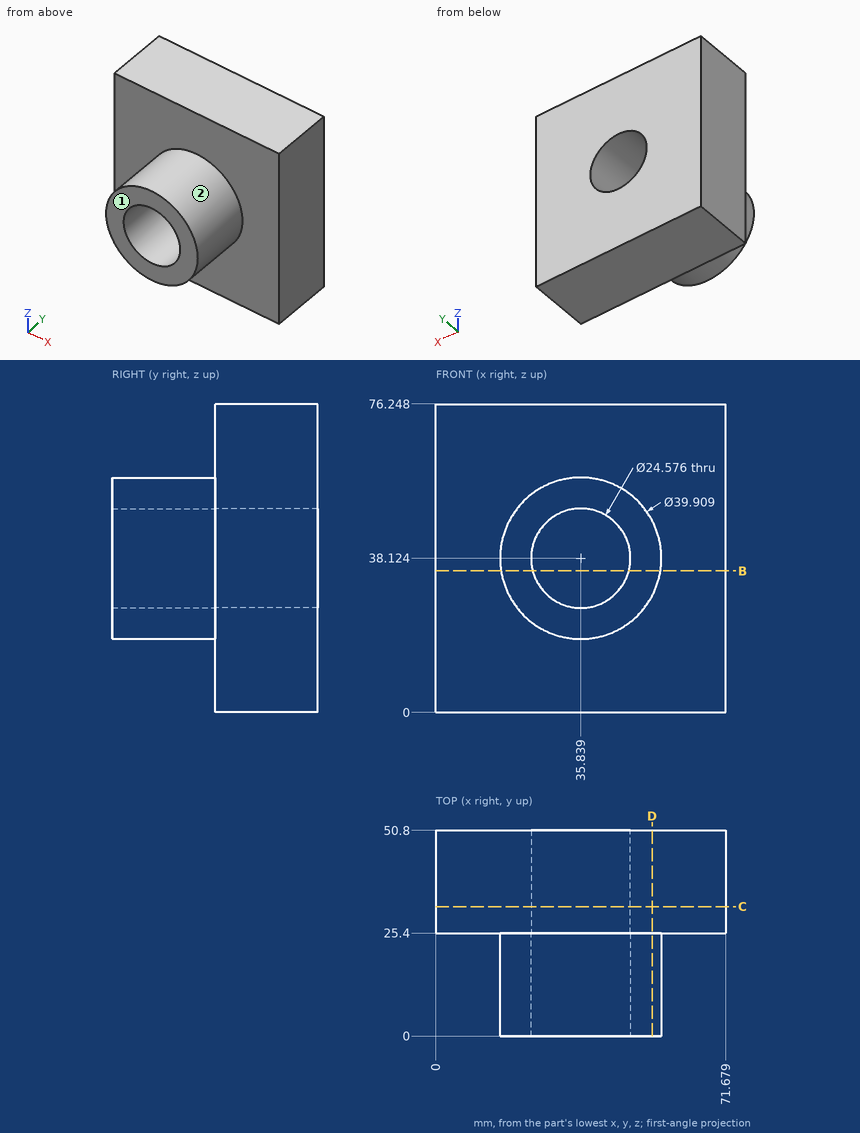
Job drawing, mm, ordinate dimensions from the low corner. One solid piece. A direction names the side the tool comes from. Round coordinates to 2 decimals unless told otherwise and drop trailing zeros. Write each loop counter-clockwise with the first axis right and the second up, starting at its lowest first coordinate (ties: lowest second). Pieces come first, ordered by that corner, then holes. Notation, with made-up numbers: (-1, 52) -> (12, 52) arc R14 ccw to (12, 60) -> close; hole circle Ø5 at (-40, 17). An arc over 180 degrees is marked (long way). Answer as a JSON object with one key per item and string values.
(1) Pin check, flat tips, straight feed: P1, Ø1, axis at y = 34.5, z = 15, coming from the -X side; P2, Ø10, axis at x = 18, z = 62, coming from the -Y side. Stop position of each tip, or through.
Reported:
{"P1": "stops at x = 0", "P2": "stops at y = 25.4"}
(2) Band-saw the part on C-C, the plane y = 32. List the corners of the cut face in (x, z), then the cut area to 3 significant figures.
Reported:
{"outline": "(0, 0) -> (71.68, 0) -> (71.68, 76.25) -> (0, 76.25) -> close; hole circle Ø24.58 at (35.84, 38.12)", "area": "4,990 mm^2"}
(3) Which spindle directions (+Z, -Z, +X, -X, +Y, -Y) get a long thin tool onto all of the face, cutting with end or side? Do the marked faces 1 and 2. Say none if no direction does.
Reported:
{"face 1": "+Z, -Z, +X, -X, -Y", "face 2": "-Y"}
(4) Probe probe 1 along Y at (x, z) = (31, 4); probe 2 along Z at (x, y) = (34, 15.5) (1 decimal); probe 3 along Z at (x, y) = (34, 39) (1 decimal). List the from-to ranges inside material, lowest first. Write a range as [from, to].
Reported:
{"probe 1": "y = [25.4, 50.8]", "probe 2": "z = [18.3, 26], [50.3, 58]", "probe 3": "z = [0, 26], [50.3, 76.2]"}
(5) Band-saw the part on B-B, the plane z = 35. List the corners of the cut face in (x, y) (1 decimal).
Reported:
{"outline": "(0, 25.4) -> (16.1, 25.4) -> (16.1, 0) -> (24, 0) -> (24, 50.8) -> (0, 50.8) -> close; (47.7, 0) -> (55.5, 0) -> (55.5, 25.4) -> (71.7, 25.4) -> (71.7, 50.8) -> (47.7, 50.8) -> close"}
(6) Band-saw the part on D-D, the plane x = 53.5. List the corners of the cut face in (y, z) (1 decimal), then the cut area to 3 significant figures.
Reported:
{"outline": "(0, 28.8) -> (25.4, 28.8) -> (25.4, 0) -> (50.8, 0) -> (50.8, 76.2) -> (25.4, 76.2) -> (25.4, 47.4) -> (0, 47.4) -> close", "area": "2,410 mm^2"}
